from build123d import *

# Parameters (mm, degrees)
SKETCH018_R         = 75.1
SKETCH018_W         = 4.8
SKETCH018_H         = 19.8
PAD018_DEPTH        = 5
CUT_PLACEMENT_ANGLE = 90


with BuildPart() as revolution:
    # Sketch019 → Revolution (revolve)
    with BuildSketch(Plane.XZ):
        with BuildLine():
            Line((-75.1, 0), (-75.1, 5))
            Line((-75.1, 5), (-70.462827, 5))
            ThreePointArc((-70.462827, 5), (-72.824338, 2.539809), (-75.1, 0))
        make_face()
    revolve(axis=Axis((0, 0, 0), (0, 0, 1)))


with BuildPart() as bowlsupport:
    # Sketch018 → Pad018 (new body)
    with BuildSketch(Plane.XY):
        Circle(SKETCH018_R)
        with Locations((-38.5, 0)):
            Rectangle(SKETCH018_W, SKETCH018_H, mode=Mode.SUBTRACT)
        with Locations((38.5, 0)):
            Rectangle(SKETCH018_W, SKETCH018_H, mode=Mode.SUBTRACT)
    extrude(amount=PAD018_DEPTH)

    # Cut: cut Revolution
    add(revolution.part, mode=Mode.SUBTRACT)


with BuildPart() as bowlsupport_1:
    # Cut placement: moved
    add(bowlsupport.part.moved(Location((0, 36, 160))).rotate(Axis((0, 36, 160), (0, 0, 1)), CUT_PLACEMENT_ANGLE))


solid = bowlsupport_1.part
Geometry check sheet. Reference: the model listing, model coordinates, mm. A direction names the side the tool comes from. Give positions to 0.01 mm unless a question says otherwise; leave off trailing zeros.
1) Draft check along X on faces 1 (the flat face through (-1, 35, 165)), 2 (the flat face through (9.9, 74, 162)). Enter one of: released by +X, released by -X, zero draft, split by the parting line, or undercut.
Results are:
face 1: zero draft
face 2: undercut
2) Tool access check on faces 3 (the flat face through (0, -4.9, 162)), 4 (the flat face through (-1, 35, 160)). Record the directions out of +Z, -Z, +X, -X, +Y, -Y that give a thin tool (end or side, any length) a straight path to the whole face; none if there is none.
Results are:
face 3: +Z, -Z
face 4: -Z, +X, -X, +Y, -Y
3) Material ranges on probe 1 along Y at (x, z) = (-6.5, 163.05); probe 2 along Y at (x, z) = (0, 160.3); probe 3 along X at (y, z) = (90, 164.6), recorded low to high.
Results are:
probe 1: y = -36.06 to -4.9, -0.1 to 72.1, 76.9 to 108.06
probe 2: y = -38.84 to -4.9, -0.1 to 72.1, 76.9 to 110.84
probe 3: x = -45.88 to 45.88
4) Cross-section at A-A (x = 4). Give the number of separate pieces and of enclosed holes in the cut face, then the cut area to 3 significant figures.
Results are:
separate pieces: 3
enclosed holes: 0
area: 679 mm2
5) Gauge pin test, flat ends, axial feed: pin 1 (2.5 mm diameter, centred on x = -2, z = 163, fed in from -Y); pin 2 (1.5 mm diameter, centred on y = 36, z = 162.5, fed in from +X); pin 3 (2 mm diameter, centred on x = 55.5, z = 162.5, fed in from -Y). Record the tip position at first contact, or that the pin passes through.
Results are:
pin 1: stops at y = -37.52
pin 2: stops at x = 73.55
pin 3: stops at y = -13.01
